Check sheet for the modelled part. Datum: model origin and axes. Units: mm. A direction names the side the tool comes from. Round coordinates to 2 decimals unless told otherwise and drop trailing zeros. Order: outer loops, then holes, each group sorted by start corner. A loop starts at its lowest first (then second) coordinate and runs counter-clockwise, first axis right, second up.
```python
from build123d import *

# Parameters (mm, degrees)
F0_R            = 38.89375
F1_DEPTH        = 7.9375
F2_R            = 26.19375
F3_DEPTH        = 0.7874
F4_R            = 2.38125
F5_DEPTH        = 10.3124
F6_R            = 2.38125
F7_R            = 3.175
F8_DEPTH        = 7.1511
F10_D           = 6.35
F10_CSINK_D     = 8.7376
F10_CSINK_ANGLE = 82
F11_R           = 3.175
F12_DEPTH       = 28.575
F13_R           = 3.175
F14_R           = 0.7874


with BuildPart() as f1:
    # F0 (on Front) → F1 (new body)
    with BuildSketch(Plane.XZ):
        Circle(F0_R)
    extrude(amount=F1_DEPTH)

    # F2 (on face) → F3 (cut)
    with BuildSketch(Plane.XZ.offset(7.9375)):
        Circle(F2_R)
    extrude(amount=-F3_DEPTH, mode=Mode.SUBTRACT)

    # F4 (on face) → F5 (join)
    with BuildSketch(Plane.XZ.offset(7.9375)):
        with Locations((0, 33.3375)):
            Circle(F4_R)
        with Locations((-28.871122, -16.66875)):
            Circle(F4_R)
        with Locations((28.871122, -16.66875)):
            Circle(F4_R)
    extrude(amount=F5_DEPTH)

    # F6
    f6_edges = [f1.edges().sort_by_distance(p)[0] for p in [
        (-2.38125, -18.2499, 33.3375),
        (26.489872, -18.2499, -16.66875),
        (-31.252372, -18.2499, -16.66875),
    ]]
    fillet(f6_edges, radius=F6_R)

    # F7 (on face) → F8 (cut, through all)
    with BuildSketch(Plane.XZ.offset(7.1501)):
        Circle(F7_R)
        with Locations((0, 12.7)):
            Circle(F7_R)
    extrude(amount=-F8_DEPTH, mode=Mode.SUBTRACT)

    # F10 (through all)
    with Locations(Plane(origin=(0, 0, 0), x_dir=(-1, 0, 0), z_dir=(0, 1, 0))):
        with Locations((0, 12.7)):
            CounterSinkHole(F10_D / 2, F10_CSINK_D / 2, counter_sink_angle=F10_CSINK_ANGLE)

    # F11 (on face) → F12 (join)
    with BuildSketch(Plane(origin=(0, 0, 0), x_dir=(-1, 0, 0), z_dir=(0, 1, 0))):
        with Locations((0, -17.4625)):
            Circle(F11_R)
    extrude(amount=F12_DEPTH)

    # F13
    f13_edges = [f1.edges().sort_by_distance(p)[0] for p in [
        (3.175, 28.575, -17.4625),
    ]]
    fillet(f13_edges, radius=F13_R)

    # F14
    f14_edges = [f1.edges().sort_by_distance(p)[0] for p in [
        (-38.89375, -7.9375, 0),
        (-38.89375, 0, 0),
    ]]
    fillet(f14_edges, radius=F14_R)


solid = f1.part
```
Item 1: Release check for a two-part mould opening along X. For faces 4 (the cylindrical face through (-30.86, -3.92, -23.67)), 5 (the flat face through (8, 0, 1)), 6 (the flat face through (0, -7.15, -5)) record: released by +X, released by -X, zero draft, split by the parting line, or undercut.
Answer:
face 4: split by the parting line
face 5: zero draft
face 6: undercut
Item 2: Access from +Z, -Z, +X, -X, +Y, -Y to the whole of each face (thin tool, end or side, straight path). Record for faces 1 (the cylindrical face through (1.5, -4.3, 9.9)), 2 (the cylindrical face through (-5.68, -7.55, -25.57)), 3 (the cylindrical face through (0.69, 12.52, -20.56)).
Answer:
face 1: +Y, -Y
face 2: -Y
face 3: +Y
Item 3: Scan lines: line 1 along Z through (x, y) = (0, -5) (3 decimals); line 2 along X through (y, z) = (-2, 12); line 3 along Y through (x, z) = (33.5, 2). Record each from-to range of solid material in increasing order.
Answer:
line 1: z = -38.894 to -3.175, 3.175 to 9.525, 15.875 to 38.894
line 2: x = -37 to -3.1, 3.1 to 37
line 3: y = -7.94 to 0
Item 4: Sectioned sample at A-A (x = 0). State how many separate pieces and enclosed holes the cut face has, and give its area (3 significant figures).
Answer:
separate pieces: 3
enclosed holes: 0
area: 707 mm2
Item 5: Sectioned sample at B-B (z = 0). Record the cut outline in (x, y) (1 decimal), and give its area (3 significant figures).
Answer:
outline: (-38.9, -7.2) arc R0.8 ccw to (-38.1, -7.9) - (-26.2, -7.9) - (-26.2, -7.2) - (-3.2, -7.2) - (-3.2, 0) - (-38.1, 0) arc R0.8 ccw to (-38.9, -0.8) - close; (3.2, -7.2) - (26.2, -7.2) - (26.2, -7.9) - (38.1, -7.9) arc R0.8 ccw to (38.9, -7.2) - (38.9, -0.8) arc R0.8 ccw to (38.1, 0) - (3.2, 0) - close
area: 530 mm2
Item 6: Go/stop test with flat-tipped pins: P1, Ø5, axis at y = 12, z = -15, coming from the -X side (3 decimals); P2, Ø12, axis at x = 19, y = 1.5, coming from the -Z side; P3, Ø8.5, axis at x = 0, z = 0, coming from the +Y side. Record where each tip stops, or that it passes through.
Answer:
P1: stops at x = -3.175
P2: stops at z = -36.5
P3: stops at y = 0
